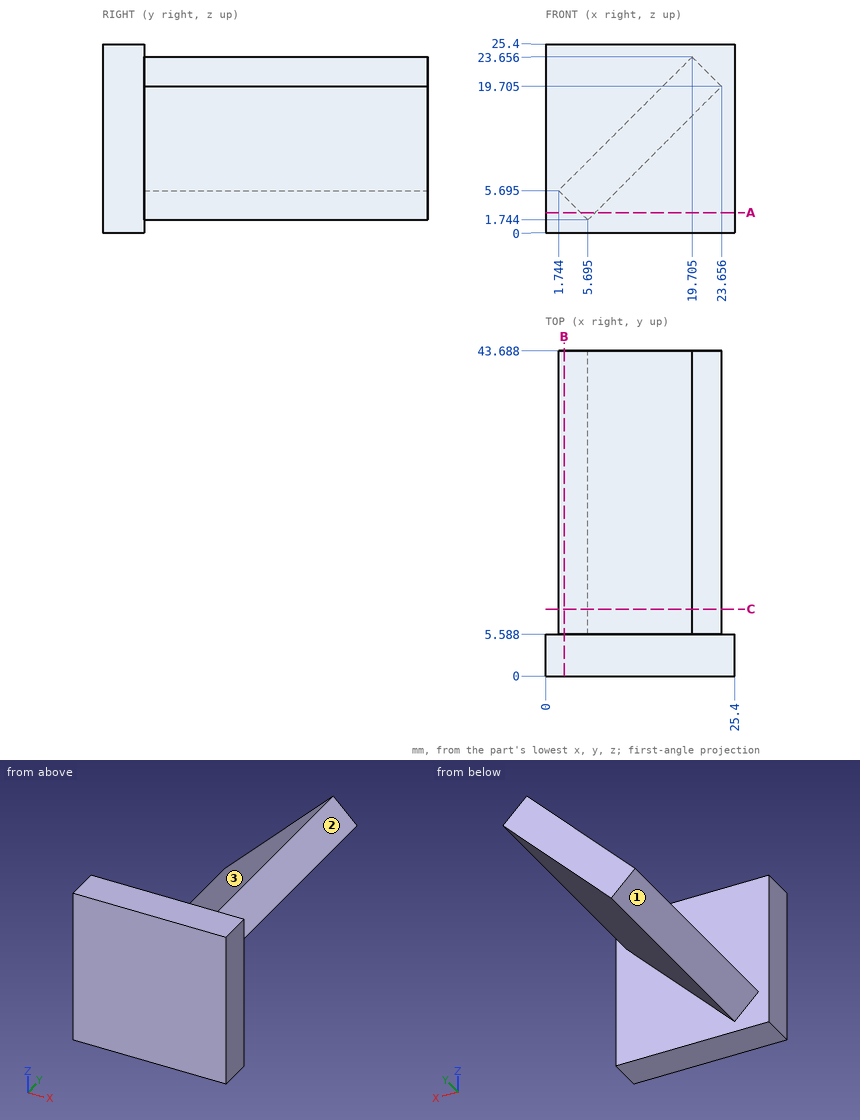
Drawing for the job (mm, zero at the part's lowest x, y, z). A direction names the side the tool comes from. Give positions to 0.01 mm unless a question says otherwise; leave off trailing zeros. Write each loop counter-clockwise with the first axis right and the second up, starting at its lowest first coordinate (ties: lowest second). Pieces come first, ordered by that corner, then holes. Notation, with made-up numbers: (-24.5, 27.5) - (-14.5, 27.5) arc R19 ccw to (-14.5, 58.5) - close; hole circle Ø7 at (32, 28.5). An arc over 180 degrees is marked (long way). Answer as CSV lines item,"result".
Q1. Drill centre lines: line 1 (Y direction, x = 1.75, z = 16); line 2 (X direction, y = 31, z = 10.25); line 3 (Z direction, x = 17.25, y = 23). Where is each one in solid material? Low to high. Write a range as from..to.
Result set:
line 1,"0..5.59"
line 2,"6.3..14.2"
line 3,"13.3..21.2"
Q2. Band-saw the part on A-A (z = 2.75). Give the cut face in (x, y).
Result set:
outline,"(0, 0) - (25.4, 0) - (25.4, 5.59) - (6.7, 5.59) - (6.7, 43.69) - (4.69, 43.69) - (4.69, 5.59) - (0, 5.59) - close"
Q3. Band-saw the part on C-C (y = 9). Give the cut face in (x, z) (1 decimal).
Result set:
outline,"(1.7, 5.7) - (5.7, 1.7) - (23.7, 19.7) - (19.7, 23.7) - close"
Q4. 3-axis set-ups, long thin cutter, end or side, ignore diameter. For the marked faces 1, 2 and 3: which of +Z, -Z, +X, -X, +Y, -Y reach the whole face in a straight line?
Result set:
face 1,"-Z, -X, +Y"
face 2,"+Z, +X, +Y"
face 3,"+Z, -X, +Y"
Q5. Band-saw the part on B-B (x = 2.5). Give the cut face in (y, z).
Result set:
outline,"(0, 0) - (5.59, 0) - (5.59, 4.94) - (43.69, 4.94) - (43.69, 6.45) - (5.59, 6.45) - (5.59, 25.4) - (0, 25.4) - close"
Q6. Flat gauge pins, fed straight in: pin 1 Ø5 at (x, z) = (9, 4) entering from -Y; pin 2 Ø1.5 at (y, z) = (10.5, 14) entering from +X; pin 3 Ø12 at (y, z) = (21.5, 9.5) entering from -X; pin 4 Ø10 at (x, y) = (18, 28) entering from -Z. Where does each tip first touch, or does it go through?
Result set:
pin 1,"y = 0"
pin 2,"x = 18.7"
pin 3,"x = 1.74"
pin 4,"z = 9.05"
